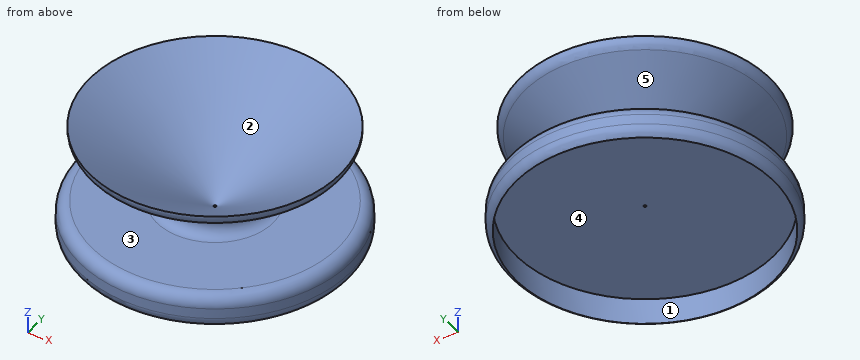
from build123d import *

# Parameters (mm, degrees)
F2_T = -2.54


# Not quite as in the source:
# - a fillet or chamfer that OpenCascade refuses, or shapes differently, is made with other operations: its cross-section is extruded or revolved along the edge and cut away or added


with BuildPart() as f1:
    # F0 (on Front) → F1 (revolve)
    with BuildSketch(Plane.XZ):
        Polygon((-8.6911804974, 13.8674174355), (0, 13.8674174355), (0, 48.0571240187), (-58.2820437849, 48.0571240187), align=None)
        Polygon((-58.0264218152, 0), (0, 0), (0, 13.8674174355), (-8.6911804974, 13.8674174355), (-58.0264218152, 13.8674174355), align=None)
    revolve(axis=Axis((0, 0, 30.9622707271), (0, 0, -1)))

    # F2
    f2_openings = [f1.faces().sort_by_distance(p)[0] for p in [
        (0, 0, 48.057124),
        (0, 0, 0),
    ]]
    offset(amount=F2_T, openings=f2_openings, kind=Kind.INTERSECTION)

    # F3: fillet of radius 5.08 on 6 edges, made by hand

    # F3_s1 → F3_t2 (revolve)
    with BuildSketch(Plane.XZ):
        with BuildLine():
            ThreePointArc((-22.1258654795, 23.1297675365), (-20.1589276546, 17.4374403683), (-25.0093265306, 13.8674174355))
            Line((-25.0093265306, 13.8674174355), (-8.6911804974, 13.8674174355))
            Line((-8.6911804974, 13.8674174355), (-22.1258654795, 23.1297675365))
        make_face()
    revolve(axis=Axis((0, 0, 13.8674174355), (0, 0, -1)))

    # F3_s3 → F3_t4 (revolve, cut)
    with BuildSketch(Plane.XZ):
        with BuildLine():
            ThreePointArc((-51.6268528261, 43.4687984471), (-53.3317173465, 45.4708576387), (-53.8071437354, 48.0571240187))
            Line((-53.8071437354, 48.0571240187), (-58.2820437849, 48.0571240187))
            Line((-58.2820437849, 48.0571240187), (-51.6268528261, 43.4687984471))
        make_face()
    revolve(axis=Axis((0, 0, 48.0571240187), (0, 0, -1)), mode=Mode.SUBTRACT)

    # F3_s5 → F3_t6 (revolve, cut)
    with BuildSketch(Plane.XZ):
        with BuildLine():
            ThreePointArc((-52.9464218152, 13.8674174355), (-56.5385242636, 12.3795198839), (-58.0264218152, 8.7874174355))
            Line((-58.0264218152, 8.7874174355), (-58.0264218152, 13.8674174355))
            Line((-58.0264218152, 13.8674174355), (-52.9464218152, 13.8674174355))
        make_face()
    revolve(axis=Axis((0, 0, 13.8674174355), (0, 0, -1)), mode=Mode.SUBTRACT)

    # F3_s7 → F3_t8 (revolve, cut)
    with BuildSketch(Plane.XZ):
        with BuildLine():
            ThreePointArc((-58.0264218152, 4.3994090512), (-57.3458308664, 1.8594090512), (-55.4864218152, 0))
            Line((-55.4864218152, 0), (-58.0264218152, 0))
            Line((-58.0264218152, 0), (-58.0264218152, 4.3994090512))
        make_face()
    revolve(axis=Axis((0, 0, 0), (0, 0, -1)), mode=Mode.SUBTRACT)


solid = f1.part
The listing builds one solid part. Answer for the finished solid, in the listing's coordinates (mm). Face numbers are marked on the shaded views. A direction names the side the tool comes from. Round coordinates to 2 decimals unless told otherwise and drop trailing zeros. Write each loop counter-clockwise with the first axis right and the second up, starting at its lowest first coordinate (ties: lowest second). Pieces come first, ordered by that corner, then holes. Notation, with made-up numbers: (63.25, -39.75) - (113.25, -39.75) arc R21 cw to (113.25, -23.75) - close; hole circle Ø8 at (85.25, 66.5). An arc over 180 degrees is marked (long way). Use a Markdown table: item, result. Add a question column.
1. A tool of negligible diameter and unlimited length cuts with its end or side. For the marked faces 1 and 2, from which of +Z, -Z, +X, -X, +Y, -Y can it reach the whole face along a straight path? Write none if from no direction.
2. Flat-ended cylindrical pins translate along their axes: P1, Ø5, axis at x = 40.5, y = -15.5, coming from the +Z side; P2, Ø1, axis at x = 35, y = -44.5, coming from the +Z side; P3, Ø3, axis at x = 39, y = 31, coming from the -Z side; P4, Ø4, axis at x = -31, z = 17.5, coming from the +Y side. Find the tip coordinate at first contact, or state that the pin passes through.
3. For a pull along X with two mould halves and no side action, classify the marked faces 3, 4 and 5 as +X half, -X half, draft (parallel to the pull), parting line (faces both ways), or undercut.
4. The part is cut by section A-A (z = 26.5). Write down the section's boundary in (x, y), and give its area (3 significant figures).
5. Consider line 1 (Y direction, x = 0, z = 4.25); line 2 (Z direction, x = 13, y = -17.5); line 3 (X direction, y = 0.5, z = 19). Determine where each line is inside the solid, lowest interval first.
Reported:
| question | item | result |
|---|---|---|
| 1 | face 1 | -Z |
| 1 | face 2 | +Z |
| 2 | P1 | z = 42.58 |
| 2 | P2 | z = 12.76 |
| 2 | P3 | z = 11.33 |
| 2 | P4 | through |
| 3 | face 3 | draft |
| 3 | face 4 | undercut |
| 3 | face 5 | parting line |
| 4 | outline | circle Ø54.03 at (0, 0); hole circle Ø45.08 at (0, 0) |
| 4 | area | 697 mm^2 |
| 5 | line 1 | -58.02 to -55.49, 55.49 to 58.02 |
| 5 | line 2 | 11.33 to 15.01, 22.89 to 25.99 |
| 5 | line 3 | -19.92 to -11.65, 11.65 to 19.92 |
